```python
from build123d import *

# Parameters (mm, degrees)
SKETCH1_W           = 68.4
SKETCH1_H           = 44.9
BOSS_EXTRUDE1_DEPTH = 10
CUT_EXTRUDE1_REACH  = 44.115
SKETCH2_R           = 1.6


with BuildPart() as part:
    # Sketch1 → Boss-Extrude1 (new body)
    with BuildSketch(Plane(origin=(0, 0, 0), x_dir=(1, 0, 0), z_dir=(0, 1, 0))):
        Rectangle(SKETCH1_W, SKETCH1_H)
    extrude(amount=BOSS_EXTRUDE1_DEPTH)

    # Sketch2 → Cut-Extrude1 (cut, up to next)
    with BuildSketch(Plane(origin=(0, 0, 0), x_dir=(1, 0, 0), z_dir=(0, 1, 0)), mode=Mode.PRIVATE) as cut_extrude1_sk1:
        with Locations(Location((30.75, 18.75, 0), (0, 0, 270))):
            Circle(SKETCH2_R)
    cut_extrude1_tool1 = extrude(cut_extrude1_sk1.sketch, amount=CUT_EXTRUDE1_REACH, mode=Mode.PRIVATE) & part.part
    # Sketch2 → Cut-Extrude1 (cut, up to next)
    with BuildSketch(Plane(origin=(0, 0, 0), x_dir=(1, 0, 0), z_dir=(0, 1, 0)), mode=Mode.PRIVATE) as cut_extrude1_sk2:
        with Locations(Location((30.75, -18.75, 0), (0, 0, 270))):
            Circle(SKETCH2_R)
    cut_extrude1_tool2 = extrude(cut_extrude1_sk2.sketch, amount=CUT_EXTRUDE1_REACH, mode=Mode.PRIVATE) & part.part
    # Sketch2 → Cut-Extrude1 (cut, up to next)
    with BuildSketch(Plane(origin=(0, 0, 0), x_dir=(1, 0, 0), z_dir=(0, 1, 0)), mode=Mode.PRIVATE) as cut_extrude1_sk3:
        with Locations(Location((-30.75, -18.75, 0), (0, 0, 270))):
            Circle(SKETCH2_R)
    cut_extrude1_tool3 = extrude(cut_extrude1_sk3.sketch, amount=CUT_EXTRUDE1_REACH, mode=Mode.PRIVATE) & part.part
    # Sketch2 → Cut-Extrude1 (cut, up to next)
    with BuildSketch(Plane(origin=(0, 0, 0), x_dir=(1, 0, 0), z_dir=(0, 1, 0)), mode=Mode.PRIVATE) as cut_extrude1_sk4:
        with Locations(Location((-30.75, 18.75, 0), (0, 0, 270))):
            Circle(SKETCH2_R)
    cut_extrude1_tool4 = extrude(cut_extrude1_sk4.sketch, amount=CUT_EXTRUDE1_REACH, mode=Mode.PRIVATE) & part.part
    add(cut_extrude1_tool1.solids().sort_by_distance((30.75, 0, -18.75))[0], mode=Mode.SUBTRACT)
    add(cut_extrude1_tool2.solids().sort_by_distance((30.75, 0, 18.75))[0], mode=Mode.SUBTRACT)
    add(cut_extrude1_tool3.solids().sort_by_distance((-30.75, 0, 18.75))[0], mode=Mode.SUBTRACT)
    add(cut_extrude1_tool4.solids().sort_by_distance((-30.75, 0, -18.75))[0], mode=Mode.SUBTRACT)


solid = part.part
```
Can you work these out from the model? Positions are in its coordinate system, mm. Give positions to 0.01 mm unless a question says otherwise; leave off trailing zeros. Loops run counter-clockwise (first coordinate to the right, second up) from the corner with the lowest first, then second, coordinate; pieces in that order, holes last. Notation, with made-up numbers: M 11,56 L 55,56 A18 cw 55,91 Z; hole C 28.25,49.25 d4. An arc over 180 degrees is marked long. One line per question, with ' | ' between items. Start each with the question number.
Q1. If we section it at B-B (x = -30.75): Please give me the cut outline in (y, z).
Q2. For pin 1 Ø5 at (x, z) = (30.75, -18.75) entering from +Y, with a flat end and sliding along its axis, tell me the tip position at first contact or that it passes through.
Q3. If we mould it in two halves opening along X, with no side actions, what happens to faces 1 (the flat face through (0, 10, 0)), 2 (the cylindrical face through (-29.67, 4.93, -19.93)), 3 (the cylindrical face through (29.78, 4.93, 17.48)), 4 (the flat face through (-34.2, 5, 0))? For each: +X half, -X half, draft (parallel to the pull), parting line (faces both ways), or undercut.
Q4. If we section it at A-A (z = -18.75): Please give me the cut outline in (x, y), plus the area to 3 significant figures.
Q5. If I drill on line 1 (X direction, y = 2, z = -18.75); line 2 (Z direction, x = -30.75, y = 5); line 3 (X direction, y = 8, z = -19.5), over which ranges is the centre line in solid material (lowest first)? Write a range as from..to.
Computed:
1) outline: M 0,-22.45 L 10,-22.45 L 10,-20.35 L 0,-20.35 Z; M 0,-17.15 L 10,-17.15 L 10,17.15 L 0,17.15 Z; M 0,20.35 L 10,20.35 L 10,22.45 L 0,22.45 Z
2) pin 1: stops at y = 10
3) face 1: draft | face 2: undercut | face 3: undercut | face 4: -X half
4) outline: M -34.2,0 L -32.35,0 L -32.35,10 L -34.2,10 Z; M -29.15,0 L 29.15,0 L 29.15,10 L -29.15,10 Z; M 32.35,0 L 34.2,0 L 34.2,10 L 32.35,10 Z | area: 620 mm²
5) line 1: x = -34.2..-32.35, -29.15..29.15, 32.35..34.2 | line 2: z = -22.45..-20.35, -17.15..17.15, 20.35..22.45 | line 3: x = -34.2..-32.16, -29.34..29.34, 32.16..34.2
